Build history of the part. All positions in model axes, mm. Face numbers are marked on the shaded views. Round coordinates to 2 decimals unless told otherwise and drop trailing zeros. Write each loop counter-clockwise with the first axis right and the second up, starting at its lowest first coordinate (ties: lowest second). Pieces come first, ordered by that corner, then holes. Notation, with made-up numbers: M 73,-14 L 127,-14 A15 ccw 127,-1 Z; hole C 65,16.25 d6. An arc over 180 degrees is marked long. Write item = value, one per line.
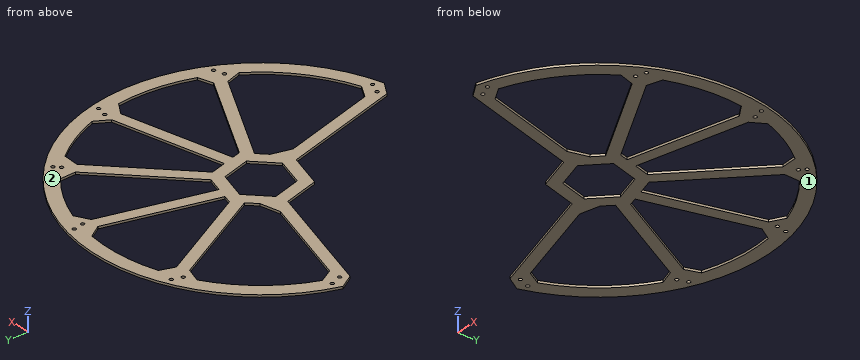
from build123d import *

# Parameters (mm, degrees)
EXTRUDE_11_DEPTH    = 2
CHAMFER_1_SIZE      = 10
CHAMFER_3_SIZE      = 10
SKETCH_4_R          = 1.52
CUT_EXTRUDE_1_DEPTH = 10


with BuildPart() as part:
    # 草图2 → 凸台-拉伸11 (new body)
    with BuildSketch(Plane.XY):
        with BuildLine():
            Line((116.986968716, -171.866279839), (116.986166566, -171.866494817))
            Line((116.986166566, -171.866494817), (146.957834859, -283.724244016))
            ThreePointArc((146.95783486, -283.724244021), (219.052953151, -31.555197901), (-33.116092969, -103.650316192))
            Line((-33.116092963, -103.650316193), (78.741656236, -133.621984487))
            Line((78.741656247, -133.621984484), (86.823548141, -163.784015655))
            Line((86.823548141, -163.784015655), (86.824011296, -163.784139757))
            Line((86.824011296, -163.784139757), (116.986968716, -171.866279839))
        make_face()
        Polygon((119.456975173, -161.769210408), (95.30929267, -155.298858383), (95.308829516, -155.298734281), (88.838353388, -131.150588624), (106.516022918, -113.472919094), (130.664168575, -119.943395221), (137.134644703, -144.091540879), align=None, mode=Mode.SUBTRACT)
        with BuildLine():
            Line((126.645296946, -169.277827092), (141.323054558, -154.60006948))
            Line((141.323054558, -154.60006948), (234.255998853, -203.48188474))
            ThreePointArc((234.255998853, -203.48188474), (200.365014055, -244.433677808), (153.509224986, -269.537128502))
            Line((153.509224986, -269.537128502), (126.645296946, -169.277827092))
        make_face(mode=Mode.SUBTRACT)
        with BuildLine():
            ThreePointArc((248.706632523, -112.641381763), (249.968706378, -154.348708565), (238.707168991, -194.526708951))
            Line((238.707168991, -194.526708951), (148.725754618, -147.19736942))
            Line((148.725754618, -147.19736942), (146.784206577, -139.951413486))
            Line((146.784206577, -139.951413486), (248.706632523, -112.641381763))
        make_face(mode=Mode.SUBTRACT)
        with BuildLine():
            ThreePointArc((-18.929686723, -97.098736021), (6.17383244, -50.2426152), (47.125895572, -16.351447355))
            Line((47.125895572, -16.351447355), (96.007676733, -109.284326822))
            Line((96.007676733, -109.284326822), (81.329397649, -123.962605906))
            Line((81.329397649, -123.962605906), (-18.929686723, -97.098736021))
        make_face(mode=Mode.SUBTRACT)
        with BuildLine():
            ThreePointArc((56.081079681, -11.900293037), (96.259335826, -0.638798731), (137.966891648, -1.901061882))
            Line((137.966891648, -1.901061882), (110.656845042, -103.823543372))
            Line((110.656845042, -103.823543372), (103.410518411, -101.881896003))
            Line((103.410518411, -101.881896003), (56.081079681, -11.900293037))
        make_face(mode=Mode.SUBTRACT)
        with BuildLine():
            ThreePointArc((147.738817906, -4.068769649), (179.372913634, -16.638491001), (206.967778767, -36.569304474))
            Line((206.967778767, -36.569304474), (133.573137745, -109.963945495))
            Line((133.573137745, -109.963945495), (120.316103305, -106.411733823))
            Line((120.316103305, -106.411733823), (147.738817906, -4.068769649))
        make_face(mode=Mode.SUBTRACT)
        with BuildLine():
            ThreePointArc((214.038825287, -43.640393577), (233.969445691, -71.235329731), (246.538975276, -102.869441968))
            Line((246.538975276, -102.869441968), (144.196016126, -130.292155223))
            Line((144.196016126, -130.292155223), (140.643866505, -117.03535236))
            Line((140.643866505, -117.03535236), (214.038825287, -43.640393577))
        make_face(mode=Mode.SUBTRACT)
    extrude(amount=-EXTRUDE_11_DEPTH)

    # 倒角1
    # the kernel refuses this chamfer: 10 mm, written as the material it adds along each edge
    with BuildSketch(Plane(origin=(246.538975276, -102.869441968, 0), x_dir=(-0.28555901452107074, 0.9583611267292487, 0), z_dir=(0, 0, -1))) as chamfer_1_piece_1:
        with BuildLine():
            Line((9.665018265, 0), (CHAMFER_1_SIZE * 0.0277867153721, -CHAMFER_1_SIZE * 0.999613874678))
            Line((CHAMFER_1_SIZE * 0.0277867153721, -CHAMFER_1_SIZE * 0.999613874678), (0, 0))
            ThreePointArc((0, 0), (4.969359021, 0.084571078), (9.665018265, 0))
        make_face()
    extrude(amount=2)
    with BuildSketch(Plane(origin=(214.038825287, -43.640393577, 0), x_dir=(-0.707106781186561, -0.707106781186534, 0), z_dir=(0, 0, -1))) as chamfer_1_piece_2:
        with BuildLine():
            Line((CHAMFER_1_SIZE, 0), (0.689672032, -9.65402706))
            ThreePointArc((0.689672032, -9.65402706), (0.269761539, -4.966357207), (0, 0))
            Line((0, 0), (CHAMFER_1_SIZE, 0))
        make_face()
    extrude(amount=2)
    with BuildSketch(Plane(origin=(238.707168991, -194.526708951, 0), x_dir=(0.38013608783902403, 0.9249305675143631, 0), z_dir=(0, 0, -1))) as chamfer_1_piece_3:
        with BuildLine():
            Line((9.685612303, 0), (CHAMFER_1_SIZE * 0.0941398773056, -CHAMFER_1_SIZE * 0.995558980423))
            Line((CHAMFER_1_SIZE * 0.0941398773056, -CHAMFER_1_SIZE * 0.995558980423), (0, 0))
            ThreePointArc((0, 0), (4.974727114, 0.084937068), (9.685612303, 0))
        make_face()
    extrude(amount=2)
    with BuildSketch(Plane(origin=(248.706632523, -112.641381763, 0), x_dir=(0.14636574749919642, -0.9892305433815727, 0), z_dir=(0, 0, -1))) as chamfer_1_piece_4:
        with BuildLine():
            Line((9.691773178, 0), (CHAMFER_1_SIZE * 0.114653249031, CHAMFER_1_SIZE * 0.99340557301))
            Line((CHAMFER_1_SIZE * 0.114653249031, CHAMFER_1_SIZE * 0.99340557301), (0, 0))
            ThreePointArc((0, 0), (4.976248684, -0.085046752), (9.691773178, 0))
        make_face()
    extrude(amount=2)
    with BuildSketch(Plane(origin=(206.967778767, -36.569304474, 0), x_dir=(-0.7556917941479319, 0.6549274099146253, 0), z_dir=(0, 0, -1))) as chamfer_1_piece_5:
        with BuildLine():
            Line((9.678628526, 0), (CHAMFER_1_SIZE * 0.0712511793936, -CHAMFER_1_SIZE * 0.997458404865))
            Line((CHAMFER_1_SIZE * 0.0712511793936, -CHAMFER_1_SIZE * 0.997458404865), (0, 0))
            ThreePointArc((0, 0), (4.972954578, 0.084812842), (9.678628526, 0))
        make_face()
    extrude(amount=2)
    with BuildSketch(Plane(origin=(147.738817906, -4.068769649, 0), x_dir=(0.9583596366559947, -0.28556401529007475, 0), z_dir=(0, 0, -1))) as chamfer_1_piece_6:
        with BuildLine():
            Line((9.665019928, 0), (CHAMFER_1_SIZE * 0.0277919314036, CHAMFER_1_SIZE * 0.999613729672))
            Line((CHAMFER_1_SIZE * 0.0277919314036, CHAMFER_1_SIZE * 0.999613729672), (0, 0))
            ThreePointArc((0, 0), (4.969359471, -0.084571108), (9.665019928, 0))
        make_face()
    extrude(amount=2)
    with BuildSketch(Plane(origin=(153.509224986, -269.537128502, 0), x_dir=(0.9450297338640432, 0.32698440652859245, 0), z_dir=(0, 0, -1))) as chamfer_1_piece_7:
        with BuildLine():
            Line((9.678629813, 0), (CHAMFER_1_SIZE * 0.071255359942, -CHAMFER_1_SIZE * 0.997458106228))
            Line((CHAMFER_1_SIZE * 0.071255359942, -CHAMFER_1_SIZE * 0.997458106228), (0, 0))
            ThreePointArc((0, 0), (4.972954909, 0.084812865), (9.678629813, 0))
        make_face()
    extrude(amount=2)
    with BuildSketch(Plane(origin=(234.255998853, -203.48188474, 0), x_dir=(-0.5077534832780394, -0.861502408713416, 0), z_dir=(0, 0, -1))) as chamfer_1_piece_8:
        with BuildLine():
            Line((9.671511766, 0), (CHAMFER_1_SIZE * 0.0483333592427, CHAMFER_1_SIZE * 0.998831260216))
            Line((CHAMFER_1_SIZE * 0.0483333592427, CHAMFER_1_SIZE * 0.998831260216), (0, 0))
            ThreePointArc((0, 0), (4.97109735, -0.08468637), (9.671511766, 0))
        make_face()
    extrude(amount=2)
    with BuildSketch(Plane(origin=(-18.929686723, -97.098736021, 0), x_dir=(0.32698155779507593, 0.9450307195334474, 0), z_dir=(0, 0, -1))) as chamfer_1_piece_9:
        with BuildLine():
            Line((9.678628888, 0), (CHAMFER_1_SIZE * 0.0712523531674, CHAMFER_1_SIZE * 0.997458321018))
            Line((CHAMFER_1_SIZE * 0.0712523531674, CHAMFER_1_SIZE * 0.997458321018), (0, 0))
            ThreePointArc((0, 0), (4.972954671, -0.084812848), (9.678628888, 0))
        make_face()
    extrude(amount=2)
    with BuildSketch(Plane(origin=(47.125895572, -16.351447355, 0), x_dir=(-0.8615033162863328, -0.5077519434011564, 0), z_dir=(0, 0, -1))) as chamfer_1_piece_10:
        with BuildLine():
            Line((9.671511206, 0), (CHAMFER_1_SIZE * 0.0483315739005, -CHAMFER_1_SIZE * 0.998831346607))
            Line((CHAMFER_1_SIZE * 0.0483315739005, -CHAMFER_1_SIZE * 0.998831346607), (0, 0))
            ThreePointArc((0, 0), (4.971097202, 0.08468636), (9.671511206, 0))
        make_face()
    extrude(amount=2)
    with BuildSketch(Plane(origin=(56.081079681, -11.900293037, 0), x_dir=(0.46552074617297745, -0.8850369680880875, 0), z_dir=(0, 0, -1))) as chamfer_1_piece_11:
        with BuildLine():
            Line((CHAMFER_1_SIZE, 0), (0.911819668, -9.642597213))
            ThreePointArc((0.911819668, -9.642597213), (0.383769224, -4.960629667), (0, 0))
            Line((0, 0), (CHAMFER_1_SIZE, 0))
        make_face()
    extrude(amount=2)
    with BuildSketch(Plane(origin=(137.966891648, -1.901061882, 0), x_dir=(-0.258819045102493, -0.9659258262890758, 0), z_dir=(0, 0, -1))) as chamfer_1_piece_12:
        with BuildLine():
            Line((CHAMFER_1_SIZE, 0), (1.111142712, 9.627865763))
            ThreePointArc((1.111142712, 9.627865763), (0.486031221, 4.953186227), (0, 0))
            Line((0, 0), (CHAMFER_1_SIZE, 0))
        make_face()
    extrude(amount=2)
    # the kernel refuses this chamfer: 10 mm, written as the material it takes off along each edge
    with BuildSketch(Plane(origin=(146.95783486, -283.724244018, 25.728190053), x_dir=(0.9662009253756813, 0.25779017010579985, 0), z_dir=(0, 0, -1))) as chamfer_1_2_piece_1:
        with BuildLine():
            Line((9.681979791, 0), (-CHAMFER_1_SIZE * 0.00106063647762, -CHAMFER_1_SIZE * 0.999999437516))
            Line((-CHAMFER_1_SIZE * 0.00106063647762, -CHAMFER_1_SIZE * 0.999999437516), (0, 0))
            ThreePointArc((0, 0), (4.980125863, 0.078072968), (9.681979791, 0))
        make_face()
    extrude(amount=53.456380107, mode=Mode.SUBTRACT)
    with BuildSketch(Plane(origin=(-33.116092966, -103.650316193, 25.728190053), x_dir=(0.25779017010579297, 0.966200925375683, 0), z_dir=(0, 0, -1))) as chamfer_1_2_piece_2:
        with BuildLine():
            Line((9.681979791, 0), (-CHAMFER_1_SIZE * 0.00106063647762, CHAMFER_1_SIZE * 0.999999437516))
            Line((-CHAMFER_1_SIZE * 0.00106063647762, CHAMFER_1_SIZE * 0.999999437516), (0, 0))
            ThreePointArc((0, 0), (4.980125863, -0.078072968), (9.681979791, 0))
        make_face()
    extrude(amount=53.456380107, mode=Mode.SUBTRACT)

    # 倒角3
    chamfer_3_edges = [part.edges().sort_by_distance(p)[0] for p in [
        (126.645296946, -169.277827092, -1),
        (81.329397649, -123.962605906, -1),
    ]]
    chamfer(chamfer_3_edges, length=CHAMFER_3_SIZE)

    # 草图4 → 切除-拉伸1 (cut)
    with BuildSketch(Plane(origin=(0, 0, -2), x_dir=(-1, 0, 0), z_dir=(0, 0, -1))):
        with Locations((-245.186502849, -106.060815296)):
            Circle(SKETCH_4_R)
        with Locations((-253.809433195, -107.539796629)):
            Circle(SKETCH_4_R)
        with Locations((-234.46368438, -203.099121031)):
            Circle(SKETCH_4_R)
        with Locations((-242.688279646, -200.179263146)):
            Circle(SKETCH_4_R)
        with Locations((-150.64247259, -270.384667581)):
            Circle(SKETCH_4_R)
        with Locations((-159.843873975, -273.784707323)):
            Circle(SKETCH_4_R)
        with Locations((-210.567284016, -40.040867037)):
            Circle(SKETCH_4_R)
        with Locations((-214.809924703, -35.79822635)):
            Circle(SKETCH_4_R)
        with Locations((-144.547335756, -5.421648203)):
            Circle(SKETCH_4_R)
        with Locations((-143.068354423, 3.201282143)):
            Circle(SKETCH_4_R)
        with Locations((-47.509030022, -16.144466672)):
            Circle(SKETCH_4_R)
        with Locations((-50.428887906, -7.919871406)):
            Circle(SKETCH_4_R)
        with Locations((19.776516528, -99.965678463)):
            Circle(SKETCH_4_R)
        with Locations(Location((23.176556271, -90.764277077, 0), (0, 0, 180))):
            Circle(SKETCH_4_R)
    extrude(amount=-CUT_EXTRUDE_1_DEPTH, mode=Mode.SUBTRACT)


solid = part.part
1. Band-saw the part on C-C (x = 188). List the corners of the cut face in (y, z), plus the area to 3 significant figures.
Responses:
outline = M -267.52,-2 L -253.45,-2 L -253.45,0 L -267.52,0 Z; M -179.15,-2 L -167.86,-2 L -167.86,0 L -179.15,0 Z; M -128.91,-2 L -118.55,-2 L -118.55,0 L -128.91,0 Z; M -69.68,-2 L -55.54,-2 L -55.54,0 L -69.68,0 Z; M -21.79,-2 L -7.72,-2 L -7.72,0 L -21.79,0 Z
area = 128 mm²
2. Band-saw the part on D-D (z = -0.5). Count the separate pieces of the cut face and the enclosed holes in it, plus the area to 3 significant figures.
Responses:
separate_pieces = 1
enclosed_holes = 21
area = 17,000 mm²
3. Probe probe 1 along X at (y, z) = (-46.5, -1.1); probe 2 along X at (y, z) = (-181, -1.65); probe 3 along Y at (x, z) = (154, -0.85). List the from-to ranges inside material, lowest first.
Responses:
probe_1 = -6.16 to 9.35, 62.98 to 74.28, 126.02 to 136.37, 197.04 to 232.14
probe_2 = 119.43 to 129.79, 191.51 to 212.99, 243.99 to 256.58
probe_3 = -279.84 to -261.58, -161.27 to -149.97, -138.02 to -127.67, -103.68 to -89.54, -8.58 to 6.66
4. Band-saw the part on B-B (y = -56). List the corners of the cut face in (x, z), plus the area to 3 significant figures.
Responses:
outline = M -12.86,-2 L 1.71,-2 L 1.71,0 L -12.86,0 Z; M 67.98,-2 L 79.28,-2 L 79.28,0 L 67.98,0 Z; M 123.47,-2 L 133.82,-2 L 133.82,0 L 123.47,0 Z; M 187.54,-2 L 201.68,-2 L 201.68,0 L 187.54,0 Z; M 224.26,-2 L 238.84,-2 L 238.84,0 L 224.26,0 Z
area = 130 mm²
5. Band-saw the part on A-A (x = -3). List the corners of the cut face in (y, z).
Responses:
outline = M -111.72,-2 L -101.37,-2 L -101.37,0 L -111.72,0 Z; M -62.85,-2 L -42.5,-2 L -42.5,0 L -62.85,0 Z
6. Flat gauge pins, fed straight in: pin 1 (2.5 mm diameter, centred on x = 214.81, y = -35.8, fed in from -Z); pin 2 (1 mm diameter, centred on x = 98, z = -1.5, fed in from +Y); pin 3 (1 mm diameter, centred on x = 153, z = -1, fed in from +Y). Where does each tip first touch, or does it go through?
Responses:
pin_1 = through
pin_2 = 11.68
pin_3 = 7.08
7. Mould opens along Z. For the marked faces 1 and 2 say: pulls with the +Z half, pulls with the -Z half, needs draft (parallel to the pull), parting line crosses it, or undercut.
Responses:
face_1 = pulls with the -Z half
face_2 = pulls with the +Z half
